Verification items for the finished model (mm, model axes). Face numbers are marked on the shaded views. Give positions to 0.01 mm unless a question says otherwise; leave off trailing zeros. Write each loop counter-clockwise with the first axis right and the second up, starting at its lowest first coordinate (ties: lowest second). Pieces come first, ordered by that corner, then holes.
Autodesk Inventor part; units mm, degrees
ref_plane "YZ Plane" through (0, 0, 0) normal (1, 0, 0) x (0, 1, 0)
ref_plane "XZ Plane" through (0, 0, 0) normal (0, 1, 0) x (-1, 0, 0)
ref_plane "XY Plane" through (0, 0, 0) normal (0, 0, 1) x (1, 0, 0)
sketch "Sketch1" plane through (0, 0, 0) normal (1, 0, 0) x (0, 1, 0)
  line L0 (0, 0) -> (822, 0)
  line L1 (822, 0) -> (822, -49.5)
  line L2 (822, -49.5) -> (0, -49.5)
  line L3 (0, -49.5) -> (0, 0)
  line L4 (822, 0) -> (815.75, 0)
  line L5 (815.75, 0) -> (815.75, -15)
  line L6 (815.75, -15) -> (822, -15)
  line L7 (822, -15) -> (822, 0)
  line L8 (822, 0) -> (782, 0)
  line L9 (782, 0) -> (782, -8)
  line L10 (782, -8) -> (822, -8)
  line L11 (822, -8) -> (822, 0)
  line L12 (856.5319, -24.75) -> (-65.1606, -24.75) construction
  line L13 (411, 165.682) -> (411, -1074.2454) construction
  line L14 (822, -49.5) -> (815.75, -49.5)
  line L15 (815.75, -49.5) -> (815.75, -34.5)
  line L16 (815.75, -34.5) -> (822, -34.5)
  line L17 (822, -34.5) -> (822, -49.5)
  line L18 (822, -49.5) -> (782, -49.5)
  line L19 (782, -49.5) -> (782, -41.5)
  line L20 (782, -41.5) -> (822, -41.5)
  line L21 (822, -41.5) -> (822, -49.5)
  line L22 (0, 0) -> (0, -49.5)
  line L23 (0, 0) -> (6.25, 0)
  line L24 (6.25, 0) -> (6.25, -15)
  line L25 (6.25, -15) -> (0, -15)
  line L26 (0, -15) -> (0, 0)
  line L27 (0, 0) -> (40, 0)
  line L28 (40, 0) -> (40, -8)
  line L29 (40, -8) -> (0, -8)
  line L30 (0, -8) -> (0, 0)
  line L31 (6.25, -34.5) -> (0, -34.5)
  line L32 (40, -41.5) -> (0, -41.5)
  line L33 (0, -49.5) -> (6.25, -49.5)
  line L34 (6.25, -49.5) -> (6.25, -34.5)
  line L35 (0, -34.5) -> (0, -49.5)
  line L36 (0, -49.5) -> (40, -49.5)
  line L37 (40, -49.5) -> (40, -41.5)
  line L38 (0, -41.5) -> (0, -49.5)
  point P0 (40, -49.5)
  point P1 (782, -49.5)
  point P2 (815.75, -41.5)
  point P3 (822, -34.5)
  point P4 (822, -15)
  point P5 (815.75, -8)
  point P6 (782, 0)
  point P7 (40, 0)
  point P8 (6.25, -8)
  point P9 (0, -15)
  point P10 (0, -34.5)
  point P11 (6.25, -41.5)
  dimension "d0" = 822
  dimension "d1" = 49.5
  dimension "d2" = 15
  dimension "d3" = 40
  dimension "d4" = 8
  dimension "d5" = 6.25
  dimension "d6" = 24.75
  dimension "d7" = 411
extrude "Extrusion1" add sketch "Sketch1" along normal blind 5 contours L0 L9 L10 L5 L6 L1 L16 L15 L20 L19 L2 L37 L32 L34 L31 L3 L25 L24 L29 L28
equation "\"d6\" = 0.5 * d1"
equation "\"d7\" = 0.5 * d0"
properties part number "Acrly_Wand_1"
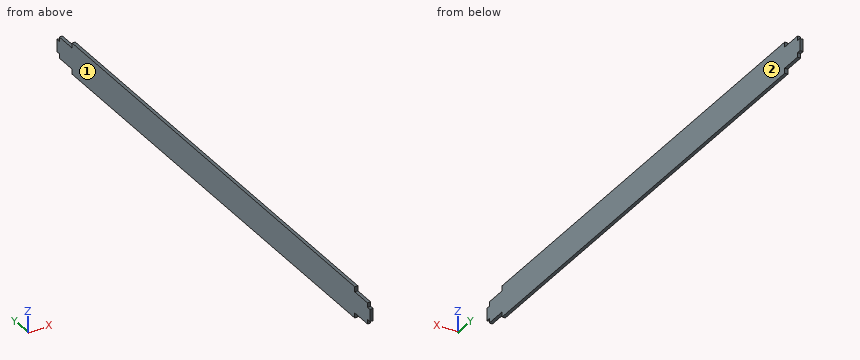
Item 1: Depth check by flat-ended pin: pin 1 (1.5 mm diameter, centred on x = 2.5, y = 804, fed in from -Z); pin 2 (1.5 mm diameter, centred on x = 3, y = 818.5, fed in from +Z); pin 3 (1.5 mm diameter, centred on x = 3, z = -13, fed in from +Y). Enter the tip coordinate at first touch or a pass-through.
Answer key:
pin 1: stops at z = -41.5
pin 2: stops at z = -15
pin 3: stops at y = 815.75
Item 2: Release check for a two-part mould opening along X. For the marked faces 1 and 2 record: released by +X, released by -X, zero draft, split by the parting line, or undercut.
Answer key:
face 1: released by -X
face 2: released by +X
Item 3: Sectioned sample at A-A on x = 3.6. Record the cut outline in (y, z).
Answer key:
outline: (0, -34.5) - (6.25, -34.5) - (6.25, -41.5) - (40, -41.5) - (40, -49.5) - (782, -49.5) - (782, -41.5) - (815.75, -41.5) - (815.75, -34.5) - (822, -34.5) - (822, -15) - (815.75, -15) - (815.75, -8) - (782, -8) - (782, 0) - (40, 0) - (40, -8) - (6.25, -8) - (6.25, -15) - (0, -15) - close
Item 4: Scan lines: line 1 along Y through (x, z) = (1.45, -2); line 2 along Y through (x, z) = (2.5, -8.5). Record each from-to range of solid material in increasing order.
Answer key:
line 1: y = 40 to 782
line 2: y = 6.25 to 815.75
